from build123d import *

# Parameters (mm, degrees)
F0_W     = 55
F0_H     = 5.6
F0_R     = 1.45
F0_R_2   = 2.775
F0_R_3   = 1.025
F1_DEPTH = 1.5
F2_DEPTH = 3.1
F3_DEPTH = 4


with BuildPart() as f1:
    # F0 (on Top) → F1 (new body)
    with BuildSketch(Plane.XY):
        Rectangle(F0_W, F0_H)
        with Locations((-24.5, 0)):
            Circle(F0_R, mode=Mode.SUBTRACT)
        with Locations((-12.5, 0)):
            Circle(F0_R_2, mode=Mode.SUBTRACT)
        with Locations((16.5, 0)):
            Circle(F0_R_2, mode=Mode.SUBTRACT)
        with Locations((24.5, 0)):
            Circle(F0_R, mode=Mode.SUBTRACT)
        with BuildLine():
            Line((-27.5, 11.775), (-27.5, 2.8))
            Line((-27.5, 2.8), (27.5, 2.8))
            Line((27.5, 2.8), (27.5, 11.775))
            ThreePointArc((27.5, 11.775), (24.278175, 19.553175), (16.5, 22.775))
            Line((16.5, 22.775), (-12.5, 22.775))
            Line((-12.5, 22.775), (-16.5, 22.775))
            ThreePointArc((-16.5, 22.775), (-24.278175, 19.553175), (-27.5, 11.775))
        make_face()
        with BuildLine():
            ThreePointArc((-9.725, 20), (-14.462221, 18.037779), (-12.5, 22.775))
            ThreePointArc((-12.5, 22.775), (-10.537779, 21.962221), (-9.725, 20))
        make_face(mode=Mode.SUBTRACT)
        with BuildLine():
            ThreePointArc((19.275, 20), (14.537779, 18.037779), (16.5, 22.775))
            ThreePointArc((16.5, 22.775), (18.462221, 21.962221), (19.275, 20))
        make_face(mode=Mode.SUBTRACT)
        with BuildLine():
            ThreePointArc((19.275, 20), (18.462221, 21.962221), (16.5, 22.775))
            ThreePointArc((16.5, 22.775), (14.537779, 18.037779), (19.275, 20))
        make_face()
        with Locations((16.5, 20)):
            Circle(F0_R_3, mode=Mode.SUBTRACT)
        with BuildLine():
            ThreePointArc((-9.725, 20), (-10.537779, 21.962221), (-12.5, 22.775))
            ThreePointArc((-12.5, 22.775), (-14.462221, 18.037779), (-9.725, 20))
        make_face()
        with Locations((-12.5, 20)):
            Circle(F0_R_3, mode=Mode.SUBTRACT)
        with Locations((16.5, 0)):
            Circle(F0_R_2)
        with Locations((16.5, 0)):
            Circle(F0_R_3, mode=Mode.SUBTRACT)
        with Locations((-12.5, 0)):
            Circle(F0_R_2)
        with Locations((-12.5, 0)):
            Circle(F0_R_3, mode=Mode.SUBTRACT)
    extrude(amount=F1_DEPTH)

    # F0 (on Top) → F2 (join)
    with BuildSketch(Plane.XY):
        Rectangle(F0_W, F0_H)
        with Locations((-24.5, 0)):
            Circle(F0_R, mode=Mode.SUBTRACT)
        with Locations((-12.5, 0)):
            Circle(F0_R_2, mode=Mode.SUBTRACT)
        with Locations((16.5, 0)):
            Circle(F0_R_2, mode=Mode.SUBTRACT)
        with Locations((24.5, 0)):
            Circle(F0_R, mode=Mode.SUBTRACT)
        with Locations((-12.5, 0)):
            Circle(F0_R_2)
        with Locations((-12.5, 0)):
            Circle(F0_R_3, mode=Mode.SUBTRACT)
        with Locations((16.5, 0)):
            Circle(F0_R_2)
        with Locations((16.5, 0)):
            Circle(F0_R_3, mode=Mode.SUBTRACT)
    extrude(amount=-F2_DEPTH)

    # F0 (on Top) → F3 (join)
    with BuildSketch(Plane.XY):
        with BuildLine():
            ThreePointArc((19.275, 20), (18.462221, 21.962221), (16.5, 22.775))
            ThreePointArc((16.5, 22.775), (14.537779, 18.037779), (19.275, 20))
        make_face()
        with Locations((16.5, 20)):
            Circle(F0_R_3, mode=Mode.SUBTRACT)
        with BuildLine():
            ThreePointArc((-9.725, 20), (-10.537779, 21.962221), (-12.5, 22.775))
            ThreePointArc((-12.5, 22.775), (-14.462221, 18.037779), (-9.725, 20))
        make_face()
        with Locations((-12.5, 20)):
            Circle(F0_R_3, mode=Mode.SUBTRACT)
        with Locations((16.5, 0)):
            Circle(F0_R_2)
        with Locations((16.5, 0)):
            Circle(F0_R_3, mode=Mode.SUBTRACT)
        with Locations((-12.5, 0)):
            Circle(F0_R_2)
        with Locations((-12.5, 0)):
            Circle(F0_R_3, mode=Mode.SUBTRACT)
    extrude(amount=F3_DEPTH)


solid = f1.part
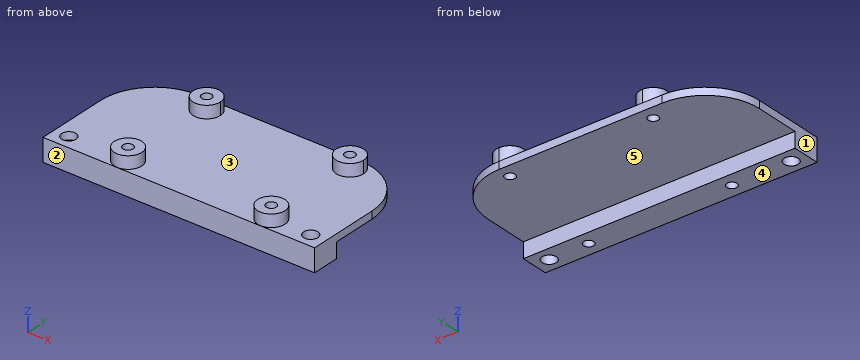
Source: CAD feature listing. Evaluate the final solid. Frame: model axes, mm. Face numbers are marked on the shaded views. A direction names the side the tool comes from. Give positions to 0.01 mm unless a question says otherwise; leave off trailing zeros. Write each loop counter-clockwise with the first axis right and the second up, starting at its lowest first coordinate (ties: lowest second). Pieces come first, ordered by that corner, then holes. Notation, with made-up numbers: (-14, 5) -> (40, 5) arc R30 cw to (40, 40) -> close; hole circle Ø1 at (-38, -40). An arc over 180 degrees is marked (long way). Write item = value, one per line.
Q1. Cut plane A-A on y = 0. Return loops of the section in (x, z) (3 decimals).
Here are the results:
outline = (-27.5, -3.1) -> (-25.95, -3.1) -> (-25.95, 1.5) -> (-27.5, 1.5) -> close; (-23.05, -3.1) -> (-13.525, -3.1) -> (-13.525, 4) -> (-15.275, 4) -> (-15.275, 1.5) -> (-23.05, 1.5) -> close; (-11.475, -3.1) -> (15.475, -3.1) -> (15.475, 4) -> (13.725, 4) -> (13.725, 1.5) -> (-9.725, 1.5) -> (-9.725, 4) -> (-11.475, 4) -> close; (17.525, -3.1) -> (23.05, -3.1) -> (23.05, 1.5) -> (19.275, 1.5) -> (19.275, 4) -> (17.525, 4) -> close; (25.95, -3.1) -> (27.5, -3.1) -> (27.5, 1.5) -> (25.95, 1.5) -> close
Q2. Mould query, pull axis Y, two halves, no side actions, for the marked faces 1, 2 and 3. Classes: +Y half, -Y half, draft (parallel to the pull), parting line (faces both ways), or undercut.
Here are the results:
face_1 = draft
face_2 = -Y half
face_3 = undercut
Q3. Line query: line 1 (Y direction, x = 16.5, z = 1) (3 decimals); line 2 (Y direction, x = -12.5, z = 2.35) (3 decimals); line 3 (Y direction, x = 16, z = 2.5). Output: solid intervals per line, ascending. Write a range as from..to.
Here are the results:
line_1 = -2.8..-1.025, 1.025..18.975, 21.025..22.775
line_2 = -2.775..-1.025, 1.025..2.775, 17.225..18.975, 21.025..22.775
line_3 = -2.73..-0.89, 0.89..2.73, 17.27..19.11, 20.89..22.73
Q4. Reachability of the marked faces 4 and 5 from +Z, -Z, +X, -X, +Y, -Y: full face, straight path, thin tool, end or side. Return the list, or none.
Here are the results:
face_4 = -Z, +X, -X, +Y, -Y
face_5 = -Z, +X, -X, +Y
Q5. Cut plane C-C on z = -0.5. Return loops of the section in (x, y) (3 decimals).
Here are the results:
outline = (-27.5, -2.8) -> (27.5, -2.8) -> (27.5, 2.8) -> (-27.5, 2.8) -> close; hole circle Ø2.9 at (-24.5, 0); hole circle Ø2.05 at (-12.5, 0); hole circle Ø2.05 at (16.5, 0); hole circle Ø2.9 at (24.5, 0)
Q6. First-contact query: pin 1 (4 mm diameter, centred on x = 19.5, y = 14, fed in from +Z); pin 2 (2.5 mm diameter, centred on x = 24.5, y = 0, fed in from -Z); pin 3 (2.5 mm diameter, centred on x = -12.5, y = 0, fed in from +Z); pin 4 (2.5 mm diameter, centred on x = 16.5, y = 20, fed in from -Z). Flat tips, straight axial feed; report the tip coordinate or a pass-through.
Here are the results:
pin_1 = 1.5
pin_2 = through
pin_3 = 4
pin_4 = 0
Q7. Cut plane B-B on z = 3.5. Return loops of the section in (x, y) (3 decimals), then the cut area to 3 significant figures.
Here are the results:
outline = circle Ø5.55 at (-12.5, 0); (-12.5, 22.775) arc R2.775 ccw (long way) to (-9.725, 20) arc R2.775 ccw to start; circle Ø5.55 at (16.5, 0); (16.5, 22.775) arc R2.775 ccw (long way) to (19.275, 20) arc R2.775 ccw to start; hole circle Ø2.05 at (-12.5, 0); hole circle Ø2.05 at (-12.5, 20); hole circle Ø2.05 at (16.5, 0); hole circle Ø2.05 at (16.5, 20)
area = 83.6 mm²
Q8. Cut plane D-D on x = -24.5. Return loops of the section in (y, z).
Here are the results:
outline = (-2.8, -3.1) -> (-1.45, -3.1) -> (-1.45, 1.5) -> (-2.8, 1.5) -> close; (1.45, -3.1) -> (2.8, -3.1) -> (2.8, 0) -> (19.32, 0) -> (19.32, 1.5) -> (1.45, 1.5) -> close
